from build123d import *

# Parameters (mm, degrees)
F0_W     = 431.8
F0_H     = 101.6
F1_DEPTH = 9.525
F2_W     = 9.525
F2_H     = 38.1
F3_DEPTH = 50.8
F4_W     = 9.525
F4_H     = 38.1
F5_DEPTH = 50.8


with BuildPart() as f1:
    # F0 (on Top) → F1 (new body)
    with BuildSketch(Plane.XY):
        Rectangle(F0_W, F0_H)
    extrude(amount=-F1_DEPTH)

    # F2 (on Front) → F3 (join, symmetric)
    with BuildSketch(Plane.XZ):
        with Locations((-163.5125, 19.05)):
            Rectangle(F2_W, F2_H)
    extrude(amount=F3_DEPTH, both=True)

    # F4 (on Front) → F5 (join, symmetric)
    with BuildSketch(Plane.XZ):
        with Locations((163.5125, 19.05)):
            Rectangle(F4_W, F4_H)
    extrude(amount=F5_DEPTH, both=True)


solid = f1.part
For this review, take the finished solid that the model builds, in its own axes (mm). A direction names the side the tool comes from. Coordinates: 2 decimals unless noted, no trailing zeros. Loops run counter-clockwise (first coordinate to the right, second up) from the corner with the lowest first, then second, coordinate; pieces in that order, holes last. Notation, with made-up numbers: (61, 58.25) - (79, 58.25) arc R31 ccw to (79, 96.25) - close; hole circle Ø2 at (44, 35). An arc over 180 degrees is marked (long way). Use a Markdown table: item, result. Add a question column.
Item 1: Insertion check: pin 1 Ø1.5 at (y, z) = (31.5, 14) entering from +X (3 decimals); pin 2 Ø1.5 at (y, z) = (-3.5, 8.5) entering from -X (3 decimals); pin 3 Ø6 at (x, z) = (-71, 1) entering from -Y; pin 4 Ø24 at (x, y) = (200.5, 4.5) entering from +Z. Each pin has a flat end and moves straight along its axis. Give the tip position at first contact, or say it passes through.
Item 2: For line 1 (X direction, y = -39.5, z = 32.5) (3 decimals); line 2 (Z direction, x = 191, y = 25.5) (3 decimals), list the stretches that pass through material, from the lowest coordinate up.
Item 3: We need section C-C (x = 119). Give the boundary of the cut face in (y, z) (3 decimals).
Item 4: We need section B-B (y = -9.5). Give the boundary of the cut face in (x, z) (3 decimals), and give its area (3 significant figures).
Item 5: Tool access review of faces 4 (the face through (192, 1, 0)), 5 (the face through (-215.9, -1, -5)), 6 (the face through (-168.275, -1, 19)), 7 (the face through (-2, 1, 0)), 8 (the face through (-1, -50.8, -3)): name each direction out of +Z, -Z, +X, -X, +Y, -Y from which nothing blocks a thin tool from reaching the whole face with its end or side.
Item 6: Mouldability with a two-part tool opening along X and no side actions: class faces 1 (the face through (215.9, -1, -5)), 2 (the face through (158.75, -1, 19)), 3 (the face through (-164, -1, 38.1)) as pulls with the +X half, pulls with the -X half, needs draft (parallel to the pull), parting line crosses it, or undercut.
Item 7: We need section A-A (z = 28). Give the boundary of the cut face in (x, y) (3 decimals), and give its area (3 significant figures).
Results list:
| question | item | result |
|---|---|---|
| 1 | pin 1 | stops at x = 168.275 |
| 1 | pin 2 | stops at x = -168.275 |
| 1 | pin 3 | stops at y = -50.8 |
| 1 | pin 4 | stops at z = 0 |
| 2 | line 1 | x = -168.275 to -158.75, 158.75 to 168.275 |
| 2 | line 2 | z = -9.525 to 0 |
| 3 | outline | (-50.8, -9.525) - (50.8, -9.525) - (50.8, 0) - (-50.8, 0) - close |
| 4 | outline | (-215.9, -9.525) - (215.9, -9.525) - (215.9, 0) - (168.275, 0) - (168.275, 38.1) - (158.75, 38.1) - (158.75, 0) - (-158.75, 0) - (-158.75, 38.1) - (-168.275, 38.1) - (-168.275, 0) - (-215.9, 0) - close |
| 4 | area | 4,840 mm^2 |
| 5 | face 4 | +Z, +X, +Y, -Y |
| 5 | face 5 | +Z, -Z, -X, +Y, -Y |
| 5 | face 6 | +Z, -X, +Y, -Y |
| 5 | face 7 | +Z, +Y, -Y |
| 5 | face 8 | +Z, -Z, +X, -X, -Y |
| 6 | face 1 | pulls with the +X half |
| 6 | face 2 | undercut |
| 6 | face 3 | needs draft |
| 7 | outline | (-168.275, -50.8) - (-158.75, -50.8) - (-158.75, 50.8) - (-168.275, 50.8) - close; (158.75, -50.8) - (168.275, -50.8) - (168.275, 50.8) - (158.75, 50.8) - close |
| 7 | area | 1,940 mm^2 |
